Verification items for this drawing (mm, ordinates from the low corner). Coordinates: 2 decimals unless noted, no trailing zeros. Write each loop counter-clockwise with the first axis right and the second up, starting at its lowest first coordinate (ties: lowest second). Pieces come first, ordered by that corner, then holes. Notation, with made-up numbers: (-30, 41.25) -> (-24, 41.25) arc R16 ccw to (-24, 55.25) -> close; hole circle Ø9 at (13, 59). An arc over 180 degrees is marked (long way). Use CSV: the item, a comma, the result in double quotes.
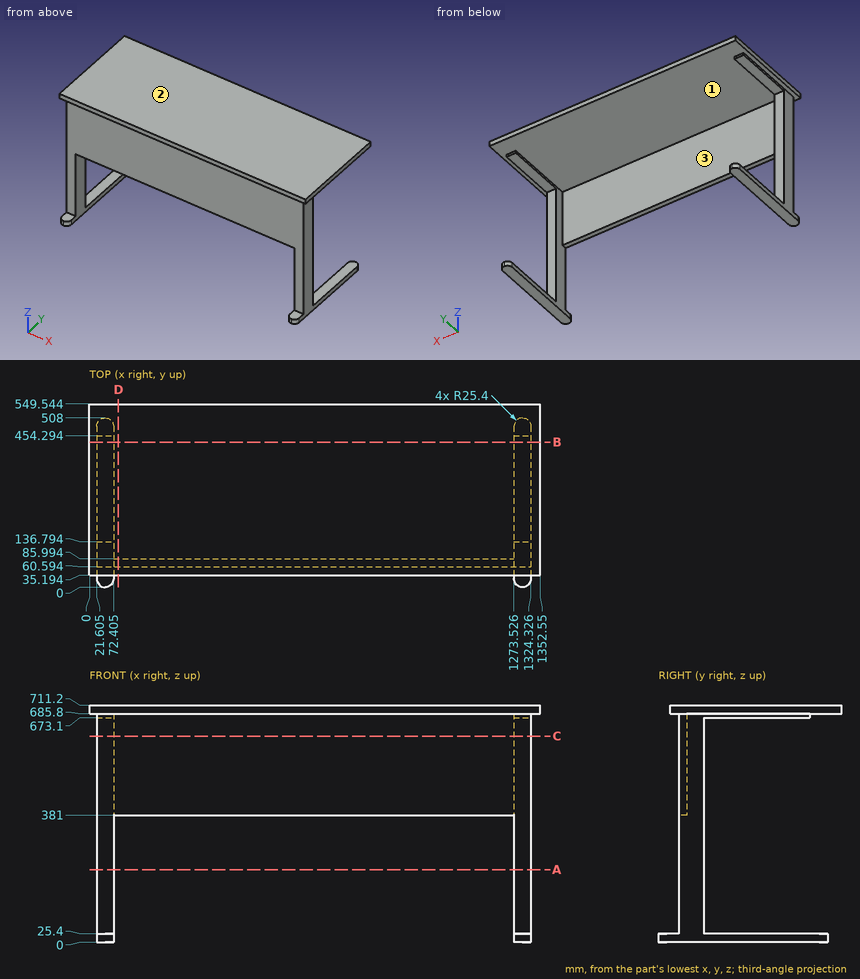
1) Scan lines: L1, parallel to Z at x = 70.5, y = 230.5; L2, parallel to Y at x = 1090.5, z = 467; L3, parallel to X at y = 430, z = 673.5 (1 decimal). Record each from-to range of solid material in increasing order.
Return value:
L1,"0 to 25.4, 673.1 to 711.2"
L2,"60.59 to 85.99"
L3,"21.6 to 72.4, 1273.5 to 1324.3"
2) Cross-section at B-B (y = 435). Give the number of separate pieces and of enclosed holes in the cut face, plus the area to 3 significant figures.
Return value:
separate pieces,"3"
enclosed holes,"0"
area,"38,200 mm2"
3) Mould release check, pull along X, two halves, no side actions. Record for the marked faces 1, 2 and 3: released by +X, released by -X, zero draft, split by the parting line, or undercut.
Return value:
face 1,"undercut"
face 2,"zero draft"
face 3,"undercut"
4) Cross-section at A-A (z = 217.5). Record the boundary of the cut face in (x, y) (1 decimal).
Return value:
outline,"(21.6, 60.6) -> (72.4, 60.6) -> (72.4, 136.8) -> (21.6, 136.8) -> close; (1273.5, 60.6) -> (1324.3, 60.6) -> (1324.3, 136.8) -> (1273.5, 136.8) -> close"
5) Cross-section at C-C (z = 618.5). Record the boundary of the cut face in (x, y) (1 decimal), plus the area to 4 significant figures.
Return value:
outline,"(21.6, 60.6) -> (1324.3, 60.6) -> (1324.3, 136.8) -> (1273.5, 136.8) -> (1273.5, 86) -> (72.4, 86) -> (72.4, 136.8) -> (21.6, 136.8) -> close"
area,"38,250 mm2"
6) Gauge pin test, flat ends, axial feed: pin 1 (4 mm diameter, centred on x = 202, z = 597, fed in from -Y); pin 2 (8 mm diameter, centred on x = 581, z = 612.5, fed in from +Y); pin 3 (10 mm diameter, centred on x = 40.5, z = 679, fed in from +Y); pin 4 (15 mm diameter, centred on x = 45.5, y = 282.5, fed in from -Z). Record the tip position at first contact, or that the pin passes through.
Return value:
pin 1,"y = 60.59"
pin 2,"y = 85.99"
pin 3,"y = 454.29"
pin 4,"z = 0"
7) Cross-section at D-D (x = 86.5). Record the boundary of the cut face in (y, z).
Return value:
outline,"(35.19, 685.8) -> (60.59, 685.8) -> (60.59, 381) -> (85.99, 381) -> (85.99, 685.8) -> (549.54, 685.8) -> (549.54, 711.2) -> (35.19, 711.2) -> close"
